from build123d import *

# Parameters (mm, degrees)
F0_R     = 4
F1_DEPTH = 20
F2_DEPTH = 15


with BuildPart() as f1:
    # F0 (on Front) → F1 (new body)
    with BuildSketch(Plane.XZ):
        with BuildLine():
            ThreePointArc((9.688615, -2.476033), (9.921848, -1.247768), (10, 0))
            ThreePointArc((10, 0), (7.968689, 6.041523), (2.7, 9.628603))
            Line((2.7, 9.628603), (2.7, 7.3))
            Line((2.7, 7.3), (-2.7, 7.3))
            Line((-2.7, 7.3), (-2.7, 9.628603))
            ThreePointArc((-2.7, 9.628603), (-8.660254, 5), (-9.688615, -2.476033))
            Line((-9.688615, -2.476033), (-7.671985, -1.311731))
            Line((-7.671985, -1.311731), (-4.971985, -5.988269))
            Line((-4.971985, -5.988269), (-6.988615, -7.15257))
            ThreePointArc((-6.988615, -7.15257), (0, -10), (6.988615, -7.15257))
            Line((6.988615, -7.15257), (4.971985, -5.988269))
            Line((4.971985, -5.988269), (7.671985, -1.311731))
            Line((7.671985, -1.311731), (9.688615, -2.476033))
        make_face()
        Circle(F0_R, mode=Mode.SUBTRACT)
        with BuildLine():
            Line((-7.671985, -1.311731), (-9.688615, -2.476033))
            ThreePointArc((-9.688615, -2.476033), (-8.660254, -5), (-6.988615, -7.15257))
            Line((-6.988615, -7.15257), (-4.971985, -5.988269))
            Line((-4.971985, -5.988269), (-7.671985, -1.311731))
        make_face()
        with BuildLine():
            Line((2.7, 7.3), (2.7, 9.628603))
            ThreePointArc((2.7, 9.628603), (0, 10), (-2.7, 9.628603))
            Line((-2.7, 9.628603), (-2.7, 7.3))
            Line((-2.7, 7.3), (2.7, 7.3))
        make_face()
        with BuildLine():
            ThreePointArc((6.988615, -7.15257), (8.660254, -5), (9.688615, -2.476033))
            Line((9.688615, -2.476033), (7.671985, -1.311731))
            Line((7.671985, -1.311731), (4.971985, -5.988269))
            Line((4.971985, -5.988269), (6.988615, -7.15257))
        make_face()
    extrude(amount=-F1_DEPTH)

    # F0 (on Front) → F2 (cut)
    with BuildSketch(Plane.XZ):
        with BuildLine():
            Line((-7.671985, -1.311731), (-9.688615, -2.476033))
            ThreePointArc((-9.688615, -2.476033), (-8.660254, -5), (-6.988615, -7.15257))
            Line((-6.988615, -7.15257), (-4.971985, -5.988269))
            Line((-4.971985, -5.988269), (-7.671985, -1.311731))
        make_face()
        with BuildLine():
            Line((2.7, 7.3), (2.7, 9.628603))
            ThreePointArc((2.7, 9.628603), (0, 10), (-2.7, 9.628603))
            Line((-2.7, 9.628603), (-2.7, 7.3))
            Line((-2.7, 7.3), (2.7, 7.3))
        make_face()
        with BuildLine():
            ThreePointArc((6.988615, -7.15257), (8.660254, -5), (9.688615, -2.476033))
            Line((9.688615, -2.476033), (7.671985, -1.311731))
            Line((7.671985, -1.311731), (4.971985, -5.988269))
            Line((4.971985, -5.988269), (6.988615, -7.15257))
        make_face()
    extrude(amount=-F2_DEPTH, mode=Mode.SUBTRACT)


solid = f1.part
Input: part model. Units: mm. Frame: model coordinates. A direction names the side the tool comes from. Round coordinates to 2 decimals unless told otherwise and drop trailing zeros. Write each loop counter-clockwise with the first axis right and the second up, starting at its lowest first coordinate (ties: lowest second). Pieces come first, ordered by that corner, then holes.
1) Ray query, L1, parallel to X at y = 15, z = 3.5; L2, parallel to X at y = 9.75, z = 1.5; L3, parallel to Z at x = 0.25, y = 17. Return the intervals inside material, ascending.
2) Reachability of faces 1 (the flat face through (5.966, 7.395, -6.562)), 2 (the flat face through (8.69, 7.4, -1.9)), 3 (the flat face through (0, 15, 9)), 4 (the flat face through (-6.303, 7.395, -3.683)) from +Z, -Z, +X, -X, +Y, -Y: full face, straight path, thin tool, end or side. Return the list, or none.
3) Draft query along X for faces 5 (the flat face through (2.7, 7, 8)), 6 (the flat face through (-0.1, 20, -4.3)), 7 (the flat face through (-5.994, 7.395, -6.579)). Return one class per face: pulls with the +X half, pulls with the -X half, needs draft (parallel to the pull), parting line crosses it, or undercut.
4) Cut plane A-A (y = 5.5). Return the cut outline in (x, z), then the cut area to 3 significant figures.
5) Cut plane D-D (x = 5.5). Return the cut outline in (y, z).
6) Contact query for flat-ended pins moving along their axis: P1, Ø4.5, axis at x = -0.5, y = 7.5, coming from the +Z side; P2, Ø3, axis at x = -1, z = 9, coming from the -Y side; P3, Ø1, axis at x = -1, z = 1.5, coming from the +Y side; P4, Ø1.9, axis at y = 7.5, z = 8.5, coming from the -X side. Output: stop coordinate, or through.
7) Cut plane C-C (z = 3). Return the cut outline in (x, y).
8) Cut plane B-B (x = 0). Return the cut outline in (y, z), then the cut area to 4 significant figures.
Geometry says:
1. L1: x = -9.37 to -1.94, 1.94 to 9.37
1. L2: x = -9.89 to -3.71, 3.71 to 9.89
1. L3: z = -10 to -3.99, 3.99 to 10
2. face 1: +X, -Y
2. face 2: -Z, -Y
2. face 3: +Z, -Y
2. face 4: -Y
3. face 5: undercut
3. face 6: needs draft
3. face 7: pulls with the -X half
4. outline: (-9.69, -2.48) - (-7.67, -1.31) - (-4.97, -5.99) - (-6.99, -7.15) arc R10 ccw to (6.99, -7.15) - (4.97, -5.99) - (7.67, -1.31) - (9.69, -2.48) arc R10 ccw to (10, 0) arc R10 ccw to (2.7, 9.63) - (2.7, 7.3) - (-2.7, 7.3) - (-2.7, 9.63) arc R10 ccw to start; hole circle Ø8 at (0, 0)
4. area: 222 mm2
5. outline: (0, -8.35) - (20, -8.35) - (20, 8.35) - (0, 8.35) - (0, -5.07) - (15, -5.07) - (15, -6.29) - (0, -6.29) - close
6. P1: stops at z = 9.63
6. P2: stops at y = 15
6. P3: passes through
6. P4: stops at x = -6.56
7. outline: (-9.54, 0) - (-2.65, 0) - (-2.65, 20) - (-9.54, 20) - close; (2.65, 0) - (9.54, 0) - (9.54, 20) - (2.65, 20) - close
8. outline: (0, -10) - (20, -10) - (20, -4) - (0, -4) - close; (0, 4) - (20, 4) - (20, 10) - (15, 10) - (15, 7.3) - (0, 7.3) - close
8. area: 199.5 mm2
